from build123d import *

# Parameters (mm, degrees)
F0_R     = 2.5
F0_W     = 8
F0_H     = 2
F1_DEPTH = 8
F2_W     = 8
F2_H     = 2.5
F3_DEPTH = 3
F4_R     = 3.99999


# Not quite as in the source:
# - a fillet or chamfer is up to 0.001 mm smaller than in the source, because OpenCascade refuses the exact size


with BuildPart() as f1:
    # F0 (on Top) → F1 (new body)
    with BuildSketch(Plane.XY):
        Polygon((-3.5, 10), (-2.5, 10), (2.5, 10), (3.5, 10), (3.5, 17), (-3.5, 17), align=None)
        with Locations((0, 13.5)):
            Circle(F0_R, mode=Mode.SUBTRACT)
        Polygon((-2.5, -10), (2.5, -10), (2.5, -5), (2.5, 10), (-2.5, 10), align=None)
        Polygon((2.5, -5), (2.5, -10), (22, -10), (22, -8), (22, -5), (19.5, -5), align=None)
        with Locations((26, -9)):
            Rectangle(F0_W, F0_H)
        Polygon((30, -8), (30, -10), (32.5, -10), (32.5, -5), (30, -5), align=None)
        Polygon((19.5, -4), (19.5, -5), (22, -5), (22, -4), (30, -4), (30, -5), (32.5, -5), (32.5, -2), (19.5, -2), align=None)
    extrude(amount=F1_DEPTH)

    # F2 (on face) → F3 (cut)
    with BuildSketch(Plane.XZ.offset(10)):
        with Locations((26, 6.75)):
            Rectangle(F2_W, F2_H)
        with Locations((26, 1.25)):
            Rectangle(F2_W, F2_H)
    extrude(amount=-F3_DEPTH, mode=Mode.SUBTRACT)

    # F4 (radius 4 in the source; OpenCascade refuses exactly that, so slightly less here)
    f4_edges = [f1.edges().sort_by_distance(p)[0] for p in [
        (-2.5, 0, 8),
        (-2.5, 0, 0),
    ]]
    fillet(f4_edges, radius=F4_R)


solid = f1.part
Source: CAD feature listing. Evaluate the final solid. Frame: model axes, mm. A direction names the side the tool comes from. Round coordinates to 2 decimals unless told otherwise and drop trailing zeros. Order: outer loops, then holes, each group sorted by start corner. A loop starts at its lowest first (then second) coordinate and runs counter-clockwise, first axis right, second up. Notation, with made-up numbers: (-34, -40) -> (4, -40) arc R20 ccw to (4, -30) -> close; hole circle Ø11 at (30.5, 57.5). An arc over 180 degrees is marked (long way). Answer as CSV lines item,"result".
Item 1: Line query: L1, parallel to Y at x = 26, z = 5; L2, parallel to Y at x = 0, z = 4; L3, parallel to Y at x = 21.5, z = 5.25. Output: solid intervals per line, ascending.
A:
L1,"-10 to -8, -4 to -2"
L2,"-10 to 11, 16 to 17"
L3,"-10 to -2"
Item 2: Pin query (flat end, axial travel): pin 1 Ø1 at (x, y) = (26, -8.5) entering from +Z; pin 2 Ø3 at (y, z) = (-8, 3.5) entering from -X; pin 3 Ø1.5 at (x, z) = (16.5, 7) entering from +Y. Return the tip coordinate at first contact, or that it passes through.
A:
pin 1,"z = 5.5"
pin 2,"x = -2.5"
pin 3,"y = -5"
Item 3: Section C-C, the plane z = 3.5. Return loops of the section in (x, y).
A:
outline,"(-3.5, 10) -> (-2.47, 10) -> (-2.47, -10) -> (32.5, -10) -> (32.5, -2) -> (19.5, -2) -> (19.5, -5) -> (2.5, -5) -> (2.5, 10) -> (3.5, 10) -> (3.5, 17) -> (-3.5, 17) -> close; hole circle Ø5 at (0, 13.5); hole (22, -8) -> (30, -8) -> (30, -4) -> (22, -4) -> close"
Item 4: Section A-A, the plane y = 13.5. Return loops of the section in (x, z).
A:
outline,"(-3.5, 0) -> (-2.5, 0) -> (-2.5, 8) -> (-3.5, 8) -> close; (2.5, 0) -> (3.5, 0) -> (3.5, 8) -> (2.5, 8) -> close"
Item 5: Pull-direction query (X, two-part tool) for faces 4 (the face through (-3, 10, 4)), 5 (the face through (30, -7, 4)), 6 (the face through (3.5, 13, 4)); classes: pulls with the +X half, pulls with the -X half, needs draft (parallel to the pull), parting line crosses it, or undercut.
A:
face 4,"needs draft"
face 5,"undercut"
face 6,"pulls with the +X half"
Item 6: Section B-B, the plane x = 26.5. Return loops of the section in (y, z).
A:
outline,"(-10, 2.5) -> (-8, 2.5) -> (-8, 5.5) -> (-10, 5.5) -> close; (-4, 0) -> (-2, 0) -> (-2, 8) -> (-4, 8) -> close"
Item 7: Reachability of faces 1 (the face through (19.5, -3, 4)), 2 (the face through (26, -8, 4)), 3 (the face through (22, -7, 4)) from +Z, -Z, +X, -X, +Y, -Y: full face, straight path, thin tool, end or side. Return the list, or none.
A:
face 1,"+Z, -Z, +Y"
face 2,"+Z, -Z"
face 3,"none"
